Here's how the part is built. I have some questions about the finished solid (model axes, mm). Face numbers are marked on the shaded views. Round coordinates to 2 decimals unless told otherwise and drop trailing zeros. Order: outer loops, then holes, each group sorted by start corner. A loop starts at its lowest first (then second) coordinate and runs counter-clockwise, first axis right, second up. Notation, with made-up numbers: (-10, 51) -> (-4, 51) arc R38 ccw to (-4, 89) -> close; hole circle Ø3 at (66.5, -5). An arc over 180 degrees is marked (long way). Use a Markdown table: item, result. Add a question column.
(1) I'm going to push flat-ended pins straight in: P1, Ø5.5, axis at x = -19, z = -2.5, coming from the -Y side; P2, Ø1, axis at x = -7.5, z = 1.5, coming from the +Y side. Where does each tip first touch, or does it pass through?
(2) I want a section at C-C, the plane y = -3.5. Please give me the cut outline in (x, z), then the cut area to 3 significant figures.
(3) I want a section at D-D, the plane z = 7.5. Please give me the cut outline in (x, y), then the cut area to 3 significant figures.
(4) I want a section at A-A, the plane z = 0. Please give me the cut outline in (x, y).
(5) Thinking about a two-plate mould opening in Z: for the marked faces 1, 2 and 3, which applies, pulls with the +Z half, pulls with the -Z half, needs draft (parallel to the pull), parting line crosses it, or undercut?
(6) If I drill on probe 1 along Z at (x, y) = (-12.7, -2); probe 2 along Z at (x, y) = (-3.5, -10.75); probe 3 along X at (y, z) = (-4.5, -5.5), over which ranges is the centre line in solid material (lowest first)?
(7) I want a section at B-B, the plane x = -12.7. Please give me the cut outline in (y, z).
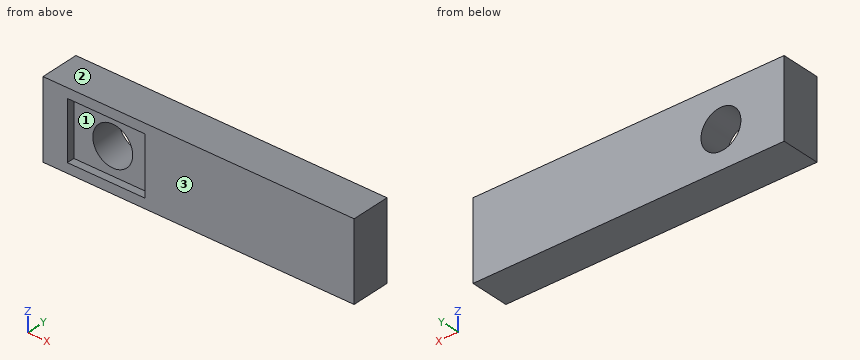
from build123d import *

# Parameters (mm, degrees)
F0_W     = 101.6
F0_H     = 25.4
F1_DEPTH = 12.7
F2_W     = 25.4
F2_H     = 19.05
F3_DEPTH = 2.54
F5_DEPTH = 25.4


with BuildPart() as f1:
    # F0 (on Front) → F1 (new body)
    with BuildSketch(Plane.XZ):
        with Locations((17.4680363059, 0.5822056818)):
            Rectangle(F0_W, F0_H)
    extrude(amount=F1_DEPTH)

    # F2 (on face) → F3 (cut)
    with BuildSketch(Plane.XZ.offset(12.7)):
        with Locations((-12.7, 0.5822056818)):
            Rectangle(F2_W, F2_H)
    extrude(amount=-F3_DEPTH, mode=Mode.SUBTRACT)

    # F4 (on face) → F5 (cut)
    with BuildSketch(Plane.XZ.offset(10.16)):
        with BuildLine():
            ThreePointArc((-19.21444736, 0), (-12.7, -6.51444736), (-6.18555264, 0))
            Line((-6.18555264, 0), (-19.21444736, 0))
        make_face()
        with BuildLine():
            Line((-19.21444736, 0), (-6.18555264, 0))
            ThreePointArc((-6.18555264, 0), (-12.7, 6.51444736), (-19.21444736, 0))
        make_face()
    extrude(amount=-F5_DEPTH, mode=Mode.SUBTRACT)


solid = f1.part
Taken from the geometry:
| question | item | result |
|---|---|---|
| 1 | P1 | stops at y = -10.16 |
| 1 | P2 | passes through |
| 2 | outline | (-33.33, -12.12) -> (68.27, -12.12) -> (68.27, 13.28) -> (-33.33, 13.28) -> close; hole circle Ø13.03 at (-12.7, 0) |
| 2 | area | 2,450 mm2 |
| 3 | outline | (-33.33, -12.7) -> (-25.4, -12.7) -> (-25.4, -10.16) -> (0, -10.16) -> (0, -12.7) -> (68.27, -12.7) -> (68.27, 0) -> (-33.33, 0) -> close |
| 3 | area | 1,230 mm2 |
| 4 | outline | (-33.33, -12.7) -> (-25.4, -12.7) -> (-25.4, -10.16) -> (-19.21, -10.16) -> (-19.21, 0) -> (-33.33, 0) -> close; (-6.19, -10.16) -> (0, -10.16) -> (0, -12.7) -> (68.27, -12.7) -> (68.27, 0) -> (-6.19, 0) -> close |
| 5 | face 1 | undercut |
| 5 | face 2 | pulls with the +Z half |
| 5 | face 3 | needs draft |
| 6 | probe 1 | z = -12.12 to -6.51, 6.51 to 13.28 |
| 6 | probe 2 | z = -12.12 to -8.94, 10.11 to 13.28 |
| 6 | probe 3 | x = -33.33 to -16.19, -9.21 to 68.27 |
| 7 | outline | (-12.7, -12.12) -> (0, -12.12) -> (0, -6.51) -> (-10.16, -6.51) -> (-10.16, -8.94) -> (-12.7, -8.94) -> close; (-12.7, 10.11) -> (-10.16, 10.11) -> (-10.16, 6.51) -> (0, 6.51) -> (0, 13.28) -> (-12.7, 13.28) -> close |
